from build123d import *

# Parameters (mm, degrees)
SKETCH_1_R          = 26
EXTRUDE_1_DEPTH     = 5
CHAMFER_1_SIZE      = 0.5
SKETCH_2_R          = 21
CUT_EXTRUDE_1_DEPTH = 10


with BuildPart() as part:
    # 草图1 → 凸台-拉伸1 (new body)
    with BuildSketch(Plane(origin=(0, 0, 0), x_dir=(1, 0, 0), z_dir=(0, 1, 0))):
        Circle(SKETCH_1_R)
    extrude(amount=EXTRUDE_1_DEPTH)

    # 倒角1
    chamfer_1_edges = [part.edges().sort_by_distance(p)[0] for p in [
        (-26, 5, 0),
    ]]
    chamfer(chamfer_1_edges, length=CHAMFER_1_SIZE)

    # 草图2 → 切除-拉伸1 (cut)
    with BuildSketch(Plane(origin=(0, 5, 0), x_dir=(1, 0, 0), z_dir=(0, 1, 0))):
        Circle(SKETCH_2_R)
    extrude(amount=-CUT_EXTRUDE_1_DEPTH, mode=Mode.SUBTRACT)


solid = part.part
Work out the finished part from the listing and answer in its coordinate system (mm). Give positions to 0.01 mm unless a question says otherwise; leave off trailing zeros. Loops run counter-clockwise (first coordinate to the right, second up) from the corner with the lowest first, then second, coordinate; pieces in that order, holes last. Notation, with made-up numbers: (-11, 57.25) - (7, 57.25) arc R19 ccw to (7, 70.25) - close; hole circle Ø1 at (72.5, 59). An arc over 180 degrees is marked (long way). Answer in a Markdown table with one row per item. Add a question column.
Q1. The part is cut by section A-A (z = 0). Determine the outline of the cut face in (x, y), and give its area (4 significant figures).
Q2. This flat-tipped pin is pushed along its axis until it touches: P1, Ø2, axis at x = -1.5, y = 4.5, coming from the +Z side. Where does it stop, or does it pass through?
Q3. Determine the mould class of faces 1 (the cylindrical face through (20.03, 2.54, -6.31)), 2 (the flat face through (1.8, 0, -21.3)), 3 (the cylindrical face through (-20.633, 2.218, 15.821)) for opening direction X: released by +X, released by -X, zero draft, split by the parting line, or undercut.
Q4. The part is cut by section B-B (x = 0). Determine the outline of the cut face in (y, z), and give its area (4 significant figures).
Q5. Consider line 1 along X through (y, z) = (1.65, 0); line 2 along X through (y, z) = (1.1, -18). Determine where each line is inside the solid, lowest interval first.
Q6. The part is cut by section C-C (y = 3.8). Determine the outline of the cut face in (x, z), and give its area (3 significant figures).
Solution:
| question | item | result |
|---|---|---|
| 1 | outline | (-26, 0) - (-21, 0) - (-21, 5) - (-25.5, 5) - (-26, 4.5) - close; (21, 0) - (26, 0) - (26, 4.5) - (25.5, 5) - (21, 5) - close |
| 1 | area | 49.75 mm² |
| 2 | P1 | stops at z = 26 |
| 3 | face 1 | undercut |
| 3 | face 2 | zero draft |
| 3 | face 3 | split by the parting line |
| 4 | outline | (0, -26) - (4.5, -26) - (5, -25.5) - (5, -21) - (0, -21) - close; (0, 21) - (5, 21) - (5, 25.5) - (4.5, 26) - (0, 26) - close |
| 4 | area | 49.75 mm² |
| 5 | line 1 | x = -26 to -21, 21 to 26 |
| 5 | line 2 | x = -18.76 to -10.82, 10.82 to 18.76 |
| 6 | outline | circle Ø52 at (0, 0); hole circle Ø42 at (0, 0) |
| 6 | area | 738 mm² |
